```python
from build123d import *

# Parameters (mm, degrees)
SKETCH_R     = 19.75
PAD_DEPTH    = 2.5
SKETCH001_R  = 13.5
PAD001_DEPTH = 27
SKETCH002_R  = 5
POCKET_DEPTH = 29.501
FILLET_R     = 1


with BuildPart() as part:
    # Sketch → Pad (new body)
    with BuildSketch(Plane.XY):
        Circle(SKETCH_R)
    extrude(amount=PAD_DEPTH)

    # Sketch001 (on Face3 of Pad) → Pad001 (join)
    with BuildSketch(Plane.XY.offset(2.5)):
        Circle(SKETCH001_R)
    extrude(amount=PAD001_DEPTH)

    # Sketch002 (on Face5 of Pad001) → Pocket (cut, through all)
    with BuildSketch(Plane.XY.offset(29.5)):
        Circle(SKETCH002_R)
    extrude(amount=-POCKET_DEPTH, mode=Mode.SUBTRACT)

    # Fillet
    fillet_edges = [part.edges().sort_by_distance(p)[0] for p in [
        (-13.5, 0, 29.5),
        (-13.5, 0, 2.5),
    ]]
    fillet(fillet_edges, radius=FILLET_R)


solid = part.part
```
Can you work these out from the model? Positions are in its coordinate system, mm. A direction names the side the tool comes from. Round coordinates to 2 decimals unless told otherwise and drop trailing zeros. Loops run counter-clockwise (first coordinate to the right, second up) from the corner with the lowest first, then second, coordinate; pieces in that order, holes last.
Item 1: Suppose I cut it at C-C, the plane z = 22. Write out the boundary of the cut face in (x, y), then the cut area to 3 significant figures.
Item 2: Please list where these lines run through material, in increasing order: L1, parallel to Y at x = 0, z = 9.5; L2, parallel to Z at x = 10, y = -11.5; L3, parallel to X at y = -2, z = 21.
Item 3: Which directions (+Z, -Z, +X, -X, +Y, -Y) give clear straight access to the entire face, cutting with the end or side of a thin tool? Please do faces 4 (the flat face through (-0.2, -5.4, 29.5)), 5 (the cylindrical face through (-2.93, -13.18, 15.82)).
Item 4: Suppose I cut it at A-A, the plane y = 0. Write out the boundary of the cut face in (x, z).
Item 5: If we mould it in two halves opening along X, with no side actions, what happens to faces 1 (the flat face through (-2, 15, 2.5)), 2 (the cylindrical face through (-14.6, 13.3, 1.2)), 3 (the cylindrical face through (-1.08, -4.88, 14.96))? For each: +X half, -X half, draft (parallel to the pull), parting line (faces both ways), or undercut.
Item 6: Suppose I cut it at D-D, the plane x = -16. Write out the boundary of the cut face in (y, z).
Item 7: Will these pins go through, and if not, where does the flat tip stop? pin 1 Ø2 at (y, z) = (-2.5, 25) entering from -X; pin 2 Ø6 at (x, z) = (0.5, 8) entering from -Y; pin 3 Ø4 at (x, y) = (8.5, -15) entering from +Z.
Reported:
1. outline: circle Ø27 at (0, 0); hole circle Ø10 at (0, 0)
1. area: 494 mm2
2. L1: y = -13.5 to -5, 5 to 13.5
2. L2: z = 0 to 2.5
2. L3: x = -13.35 to -4.58, 4.58 to 13.35
3. face 4: +Z, +X, -X, +Y, -Y
3. face 5: +Z
4. outline: (-19.75, 0) - (-5, 0) - (-5, 29.5) - (-12.5, 29.5) arc R1 ccw to (-13.5, 28.5) - (-13.5, 3.5) arc R1 cw to (-14.5, 2.5) - (-19.75, 2.5) - close; (5, 0) - (19.75, 0) - (19.75, 2.5) - (14.5, 2.5) arc R1 cw to (13.5, 3.5) - (13.5, 28.5) arc R1 ccw to (12.5, 29.5) - (5, 29.5) - close
5. face 1: draft
5. face 2: parting line
5. face 3: undercut
6. outline: (-11.58, 0) - (11.58, 0) - (11.58, 2.5) - (-11.58, 2.5) - close
7. pin 1: stops at x = -13.42
7. pin 2: stops at y = -13.5
7. pin 3: stops at z = 2.5
